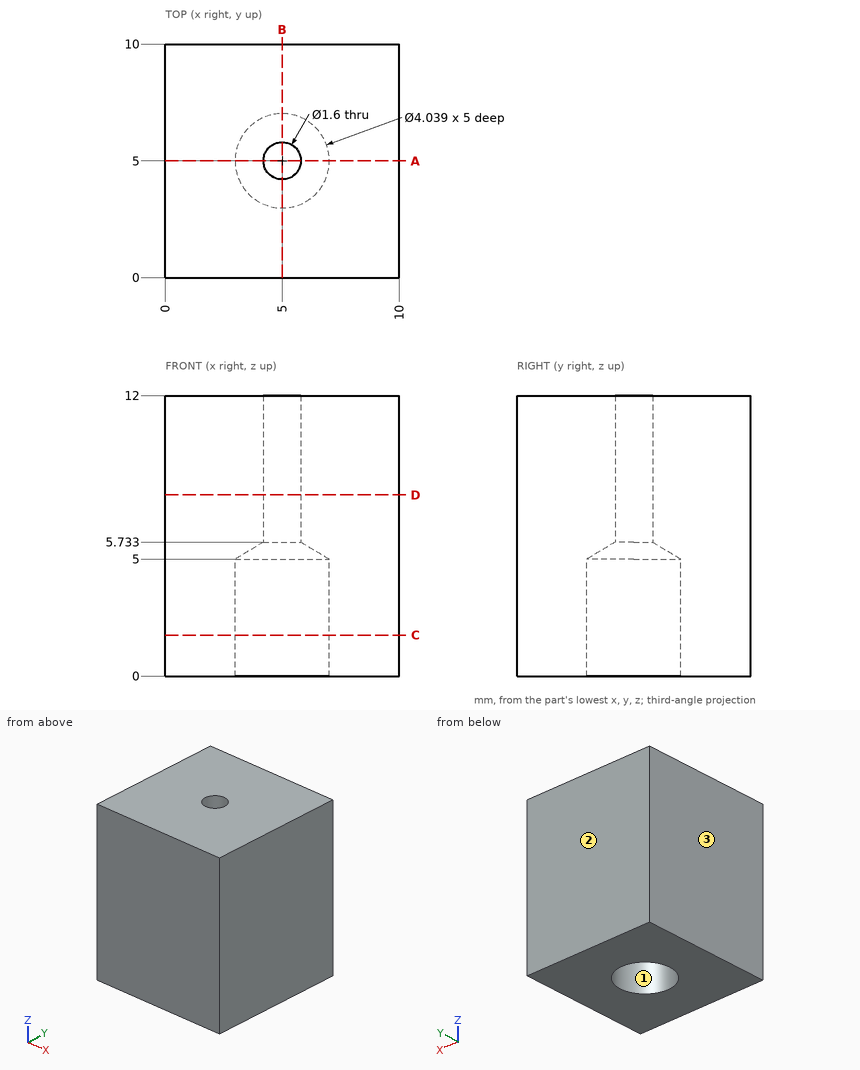
Answer from the drawing. Dimensions are ordinates in mm from the lowest x, y and z of the part. Give positions to 0.01 mm unless a question says otherwise; leave off trailing zeros. Order: outer loops, then holes, each group sorted by start corner. A loop starts at its lowest first (then second) coordinate and runs counter-clockwise, first axis right, second up. Notation, with made-up numbers: (73.25, -8) - (86.25, -8) arc R30 ccw to (86.25, 23) - close; hole circle Ø9 at (-20.75, 16). An arc over 180 degrees is marked (long way). Use one line per item in the form item = value.
1) Consider probe 1 along X at (y, z) = (5, 7.5); probe 2 along X at (y, z) = (4.75, 0.75). Determine where each line is inside the solid, lowest interval first. Write a range as [from, to].
Verdict:
probe_1 = [0, 4.2], [5.8, 10]
probe_2 = [0, 3], [7, 10]
2) Find section A-A on y = 5. Determine the outline of the cut face in (x, z).
Verdict:
outline = (0, 0) - (2.98, 0) - (2.98, 5) - (4.2, 5.73) - (4.2, 12) - (0, 12) - close; (5.8, 5.73) - (7.02, 5) - (7.02, 0) - (10, 0) - (10, 12) - (5.8, 12) - close
3) The mould has two halves that part along Y. Classify the marked faces 1, 2 and 3: released by +Y, released by -Y, zero draft, split by the parting line, or undercut.
Verdict:
face_1 = undercut
face_2 = released by +Y
face_3 = zero draft
4) Find section C-C on z = 1.75. Determine the outline of the cut face in (x, y).
Verdict:
outline = (0, 0) - (10, 0) - (10, 10) - (0, 10) - close; hole circle Ø4.04 at (5, 5)
5) Find section D-D on z = 7.75. Determine the outline of the cut face in (x, y).
Verdict:
outline = (0, 0) - (10, 0) - (10, 10) - (0, 10) - close; hole circle Ø1.6 at (5, 5)
6) Each of these flat-tipped pins is pushed along its axis until it touches: pin 1 (3 mm diameter, centred on x = 5, y = 5, fed in from -Z); pin 2 (2 mm diameter, centred on x = 5, y = 5, fed in from -Z). Where does it stop, or does it pass through?
Verdict:
pin_1 = 5.31
pin_2 = 5.61
